from build123d import *

# Parameters (mm, degrees)
F0_R      = 55
F1_DEPTH  = 4
F2_R      = 22.1
F3_DEPTH  = 2
F4_R      = 25.3
F4_R_2    = 22.1
F5_DEPTH  = 1.55
F6_R      = 28
F6_R_2    = 25.3
F7_DEPTH  = 1
F8_R      = 5
F9_DEPTH  = 25
F11_DEPTH = 1
F12_R     = 1.45
F13_DEPTH = 25
F14_R     = 1.45
F15_DEPTH = 25


with BuildPart() as f1:
    # F0 (on Top) → F1 (new body)
    with BuildSketch(Plane.XY):
        Circle(F0_R)
    extrude(amount=F1_DEPTH)

    # F2 (on face) → F3 (cut)
    with BuildSketch(Plane.XY.offset(4)):
        with Locations((27, 0)):
            Circle(F2_R)
    extrude(amount=-F3_DEPTH, mode=Mode.SUBTRACT)

    # F4 (on face) → F5 (cut)
    with BuildSketch(Plane.XY.offset(4)):
        with Locations((27, 0)):
            Circle(F4_R)
        with Locations((27, 0)):
            Circle(F4_R_2, mode=Mode.SUBTRACT)
    extrude(amount=-F5_DEPTH, mode=Mode.SUBTRACT)

    # F6 (on face) → F7 (join)
    with BuildSketch(Plane.XY.offset(4)):
        with Locations((27, 0)):
            Circle(F6_R)
        with Locations((27, 0)):
            Circle(F6_R_2, mode=Mode.SUBTRACT)
    extrude(amount=F7_DEPTH)

    # F8 (on face) → F9 (cut)
    with BuildSketch(Plane.XY.offset(2)):
        with Locations((12, 0)):
            Circle(F8_R)
    extrude(amount=-F9_DEPTH, mode=Mode.SUBTRACT)

    # F10 (on face) → F11 (join)
    with BuildSketch(Plane.XY.offset(4)):
        with BuildLine():
            ThreePointArc((10.8848586854, -22.8976466129), (7.2010101268, -19.7989898732), (4.1023533871, -16.1151413146))
            ThreePointArc((4.1023533871, -16.1151413146), (2.9583694397, -24.0416305603), (10.8848586854, -22.8976466129))
        make_face()
        with BuildLine():
            ThreePointArc((10.8848586854, 22.8976466129), (2.9583694397, 24.0416305603), (4.1023533871, 16.1151413146))
            ThreePointArc((4.1023533871, 16.1151413146), (7.2010101268, 19.7989898732), (10.8848586854, 22.8976466129))
        make_face()
        with BuildLine():
            ThreePointArc((49.8976466129, -16.1151413146), (46.7989898732, -19.7989898732), (43.1151413146, -22.8976466129))
            ThreePointArc((43.1151413146, -22.8976466129), (45.5447053375, -25.105329645), (48.8197581332, -25.3304404978))
            ThreePointArc((48.8197581332, -25.3304404978), (50.4964850216, -21.7969034605), (51.917853321, -18.1531404043))
            ThreePointArc((51.917853321, -18.1531404043), (51.0570972643, -16.9860974117), (49.8976466129, -16.1151413146))
        make_face()
        with BuildLine():
            ThreePointArc((48.8197581332, 25.3304404978), (45.5447053375, 25.105329645), (43.1151413146, 22.8976466129))
            ThreePointArc((43.1151413146, 22.8976466129), (46.7989898732, 19.7989898732), (49.8976466129, 16.1151413146))
            ThreePointArc((49.8976466129, 16.1151413146), (51.0570972643, 16.9860974117), (51.917853321, 18.1531404043))
            ThreePointArc((51.917853321, 18.1531404043), (50.4964850216, 21.7969034605), (48.8197581332, 25.3304404978))
        make_face()
    extrude(amount=F11_DEPTH)

    # F12 (on face) → F13 (cut)
    with BuildSketch(Plane.XY.offset(5)):
        with Locations((6.4939033456, 20.5060966544)):
            Circle(F12_R)
        with Locations((47.5060966544, 20.5060966544)):
            Circle(F12_R)
        with Locations((47.5060966544, -20.5060966544)):
            Circle(F12_R)
        with Locations((6.4939033456, -20.5060966544)):
            Circle(F12_R)
    extrude(amount=-F13_DEPTH, mode=Mode.SUBTRACT)

    # F14 (on face) → F15 (cut)
    with BuildSketch(Plane.XY.offset(4)):
        with Locations((0, 45)):
            Circle(F14_R)
        with Locations((-45, 0)):
            Circle(F14_R)
        with Locations((0, -45)):
            Circle(F14_R)
    extrude(amount=-F15_DEPTH, mode=Mode.SUBTRACT)


solid = f1.part
Can you work these out from the model? Positions are in its coordinate system, mm. A direction names the side the tool comes from. Coordinates: 2 decimals unless noted, no trailing zeros. Order: outer loops, then holes, each group sorted by start corner. A loop starts at its lowest first (then second) coordinate and runs counter-clockwise, first axis right, second up. Notation, with made-up numbers: (-10, -32.75) -> (34, -32.75) arc R36 cw to (34, 6.25) -> close; hole circle Ø6 at (11, 47.5). An arc over 180 degrees is marked (long way). Use one line per item in the form item = value.
Q1. Imagine slicing it at C-C, the plane x = 26. List the corners of the cut face in (y, z) for me.
From the geometry:
outline = (-48.47, 0) -> (48.47, 0) -> (48.47, 4) -> (27.98, 4) -> (27.98, 5) -> (25.28, 5) -> (25.28, 2.45) -> (22.08, 2.45) -> (22.08, 2) -> (-22.08, 2) -> (-22.08, 2.45) -> (-25.28, 2.45) -> (-25.28, 5) -> (-27.98, 5) -> (-27.98, 4) -> (-48.47, 4) -> close
Q2. Which directions (+Z, -Z, +X, -X, +Y, -Y) give clear straight access to the entire face, cutting with the end or side of a thin tool? Please do faces 5 (the face through (-1, 1, 0)), 6 (the face through (-46.45, 0.06, 2.03)), 7 (the face through (6.92, -15.39, 3.71)), 8 (the face through (26.8, -28, 4.5)), 9 (the face through (27.2, 28, 4.5)).
From the geometry:
face_5 = -Z, +X, -X, +Y, -Y
face_6 = +Z, -Z
face_7 = +Z
face_8 = +Z, -Y
face_9 = +Z, +Y
Q3. Imagine slicing it at D-D, the plane y = 37.5. List the corners of the cut face in (x, z) for me.
From the geometry:
outline = (-40.23, 0) -> (40.23, 0) -> (40.23, 4) -> (-40.23, 4) -> close
Q4. I need wall thicknesses on L1, parallel to Y at x = 0, z = 3; L2, parallel to Z at x = -26.5, y = 24; L3, parallel to Y at x = 20, z = 4.1. Which ranges of each line are inside material? Lowest first, please.
From the geometry:
L1 = -55 to -46.45, -43.55 to 43.55, 46.45 to 55
L2 = 0 to 4
L3 = -27.11 to -24.31, 24.31 to 27.11
Q5. Will these pins go through, and if not, where does the flat tip stop? P1, Ø9, axis at x = 12, y = 0, coming from the +Z side; P2, Ø1.5, axis at y = 21, z = 1.5, coming from the -X side; P3, Ø1.5, axis at x = 23.5, z = 1, coming from the -Y side; P4, Ø1.5, axis at x = -20.5, z = 2.5, coming from the -Y side.
From the geometry:
P1 = through
P2 = -51.14
P3 = -50.07
P4 = -51.33
Q6. Imagine slicing it at A-A, the plane y = -45. List the corners of the cut face in (x, z) for me, then the cut area to 3 significant figures.
From the geometry:
outline = (-31.62, 0) -> (-1.45, 0) -> (-1.45, 4) -> (-31.62, 4) -> close; (1.45, 0) -> (31.62, 0) -> (31.62, 4) -> (1.45, 4) -> close
area = 241 mm²
Q7. We'd pull the mould along X, two halves only. Please class faces 1 (the face through (45.588, 25.123, 4.493)), 2 (the face through (0.669, -46.286, 2.028)), 3 (the face through (12, 21, 5)), 4 (the face through (55, -0.2, 4.5)): released by +X, released by -X, zero draft, split by the parting line, or undercut.
From the geometry:
face_1 = undercut
face_2 = undercut
face_3 = zero draft
face_4 = released by +X
